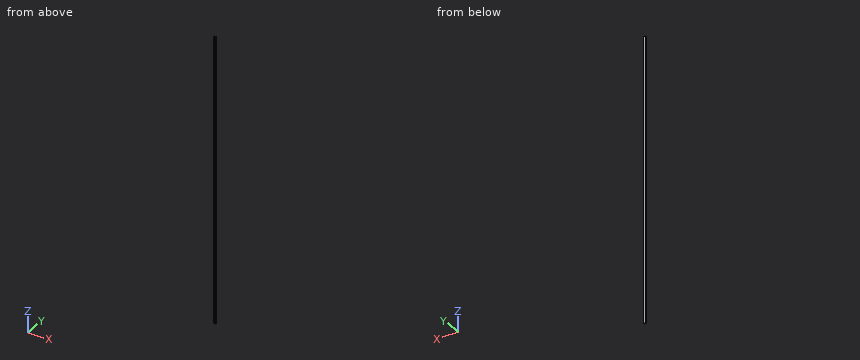
from build123d import *

# Parameters (mm, degrees)
EXTRUDE_1_DEPTH = 1000


with BuildPart() as part:
    # 草图1 → 拉伸1 (new body)
    with BuildSketch(Plane.XY):
        with BuildLine():
            Line((3.719845542, 85.778219074), (3.277947439, 86.992324134))
            ThreePointArc((3.277947439, 86.992324134), (3.2496964, 87.119756335), (3.255389873, 87.250158295))
            Line((3.255389873, 87.250158295), (3.67294288, 89.618219074))
            Line((3.67294288, 89.618219074), (3.17294288, 89.618219074))
            ThreePointArc((3.17294288, 89.618219074), (3.102232202, 89.647508396), (3.07294288, 89.718219074))
            Line((3.07294288, 89.718219074), (3.07294288, 89.918219074))
            ThreePointArc((3.07294288, 89.918219074), (3.131521524, 90.05964043), (3.27294288, 90.118219074))
            Line((3.27294288, 90.118219074), (10.07294288, 90.118219074))
            ThreePointArc((10.07294288, 90.118219074), (10.214364237, 90.05964043), (10.27294288, 89.918219074))
            Line((10.27294288, 89.918219074), (10.27294288, 89.718219074))
            ThreePointArc((10.27294288, 89.718219074), (10.243653558, 89.647508396), (10.17294288, 89.618219074))
            Line((10.17294288, 89.618219074), (9.67294288, 89.618219074))
            Line((9.67294288, 89.618219074), (10.090495888, 87.250158295))
            ThreePointArc((10.090495888, 87.250158295), (10.09618936, 87.119756335), (10.067938321, 86.992324134))
            Line((10.067938321, 86.992324134), (9.626040218, 85.778219074))
            ThreePointArc((9.626040218, 85.778219074), (9.320291197, 85.635645964), (9.177718087, 85.941394985))
            Line((9.177718087, 85.941394985), (9.596882624, 87.093040086))
            ThreePointArc((9.596882624, 87.093040086), (9.602532832, 87.118526526), (9.601394137, 87.144606918))
            Line((9.601394137, 87.144606918), (9.165229574, 89.618219074))
            Line((9.165229574, 89.618219074), (4.180656186, 89.618219074))
            Line((4.180656186, 89.618219074), (3.744491623, 87.144606918))
            ThreePointArc((3.744491623, 87.144606918), (3.743352929, 87.118526526), (3.749003137, 87.093040086))
            Line((3.749003137, 87.093040086), (4.168167674, 85.941394985))
            ThreePointArc((4.168167674, 85.941394985), (4.025594564, 85.635645964), (3.719845542, 85.778219074))
        make_face()
    extrude(amount=EXTRUDE_1_DEPTH)


solid = part.part
Model file for the job. Use its own axes, mm. Give positions to 0.01 mm unless a question says otherwise; leave off trailing zeros. Write each loop counter-clockwise with the first axis right and the second up, starting at its lowest first coordinate (ties: lowest second). Pieces come first, ordered by that corner, then holes. Notation, with made-up numbers: M -34,-1 L -7,-1 A29 ccw -7,23 Z; hole C 21.25,-28.5 d11. An arc over 180 degrees is marked long. One line per item, written item: value. Start each with the question number.
Q1. Saw through at B-B, the plane x = 7. Write the cut outline in (y, z).
Q2. Probe probe 1 along X at (y, z) = (89.1, 71); probe 2 along X at (y, z) = (88.55, 321.5); probe 3 along Y at (x, z) = (6.25, 692.5). List the from-to ranges inside material, lowest first. Write a range as [from, to].
Q3. Saw through at A-A, the plane z = 95.5. Write the cut outline in (x, y), plus the area to 3 significant figures.
Q4. Drop flat-ended pins along their axis: pin 1 Ø1.5 at (y, z) = (89.5, 504.5) entering from +X; pin 2 Ø1 at (x, y) = (7, 87) entering from -Z; pin 3 Ø1.5 at (x, z) = (6, 541) entering from -Y. Give the stop position or say it passes through.
Output values:
1. outline: M 89.62,0 L 90.12,0 L 90.12,1000 L 89.62,1000 Z
2. probe 1: x = [3.58, 4.09], [9.26, 9.76]
2. probe 2: x = [3.48, 3.99], [9.35, 9.86]
2. probe 3: y = [89.62, 90.12]
3. outline: M 3.07,89.72 A0.1 ccw 3.17,89.62 L 3.67,89.62 L 3.26,87.25 A0.5 ccw 3.28,86.99 L 3.72,85.78 A0.24 ccw 4.17,85.94 L 3.75,87.09 A0.1 cw 3.74,87.14 L 4.18,89.62 L 9.17,89.62 L 9.6,87.14 A0.1 cw 9.6,87.09 L 9.18,85.94 A0.24 ccw 9.63,85.78 L 10.07,86.99 A0.5 ccw 10.09,87.25 L 9.67,89.62 L 10.17,89.62 A0.1 ccw 10.27,89.72 L 10.27,89.92 A0.2 ccw 10.07,90.12 L 3.27,90.12 A0.2 ccw 3.07,89.92 Z
3. area: 7.57 mm²
4. pin 1: stops at x = 10.27
4. pin 2: passes through
4. pin 3: stops at y = 89.62
